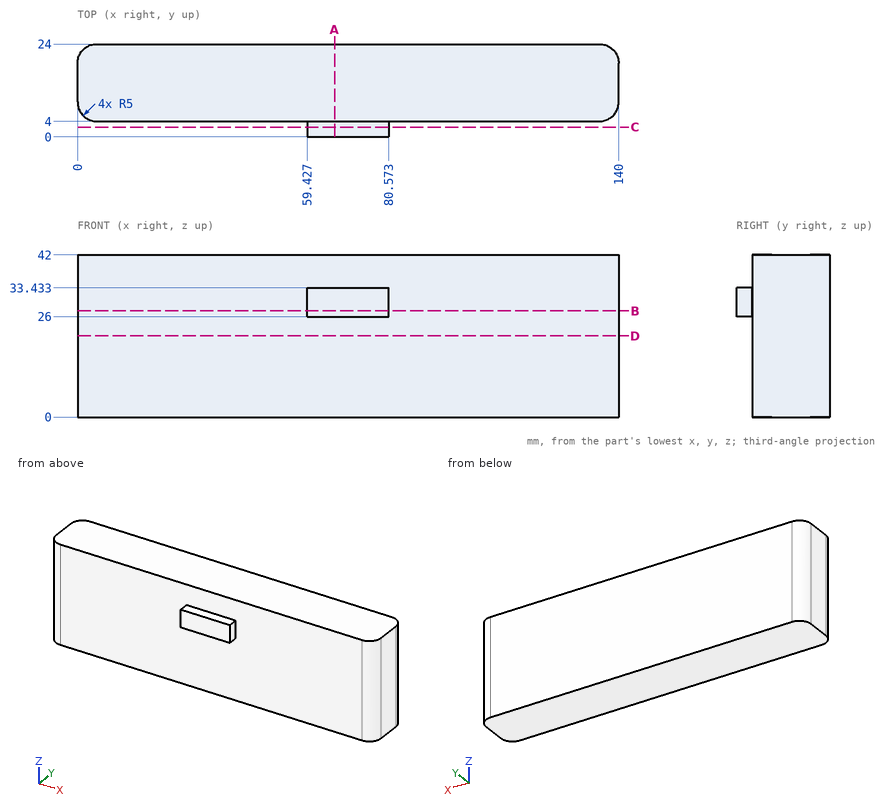
For this review, use the dimensioned drawing (mm, ordinates from the lowest corner) and the shaded views. Give positions to 0.01 mm unless a question says otherwise; leave off trailing zeros. Write each loop counter-clockwise with the first axis right and the second up, starting at its lowest first coordinate (ties: lowest second). Pieces come first, ordered by that corner, then holes. Notation, with made-up numbers: M 13,87 L 62,87 A15 cw 62,99 Z; hole C -34,42.5 d2. An arc over 180 degrees is marked long. Answer as a JSON object with one key per item and string values. Group by question number.
1) Clearance check with flat-ended pins moving along their axes: pin 1 Ø10 at (x, z) = (75, 7) entering from -Y; pin 2 Ø2 at (x, y) = (69, 2) entering from +Z; pin 3 Ø4.5 at (y, z) = (2.5, 30) entering from -X (1 decimal). State where each tip first meets the part, or that it passes through.
2) We need section D-D (z = 21). Give the boundary of the cut face in (x, y).
3) We need section A-A (x = 66.5). Give the boundary of the cut face in (y, z).
4) We need section C-C (y = 2.5). Give the boundary of the cut face in (x, z).
5) For line 1 along Y through (x, z) = (48.5, 19); line 2 along X through (y, z) = (8.5, 23.5) (1 decimal); line 3 along X through (y, z) = (4.5, 24.5) (1 decimal), list the stretches that pass through material, from the lowest coordinate up.
6) We need section B-B (z = 27.5). Give the boundary of the cut face in (x, y).
Answer key:
{
 "1": {"pin 1": "stops at y = 4", "pin 2": "stops at z = 33.43", "pin 3": "stops at x = 2.4"},
 "2": {"outline": "M 0,9 A5 ccw 5,4 L 135,4 A5 ccw 140,9 L 140,19 A5 ccw 135,24 L 5,24 A5 ccw 0,19 Z"},
 "3": {"outline": "M 0,26 L 4,26 L 4,0 L 24,0 L 24,42 L 4,42 L 4,33.43 L 0,33.43 Z"},
 "4": {"outline": "M 59.43,26 L 80.57,26 L 80.57,33.43 L 59.43,33.43 Z"},
 "5": {"line 1": "y = 4 to 24", "line 2": "x = 0 to 140", "line 3": "x = 2.8 to 137.2"},
 "6": {"outline": "M 0,9 A5 ccw 5,4 L 59.43,4 L 59.43,0 L 80.57,0 L 80.57,4 L 135,4 A5 ccw 140,9 L 140,19 A5 ccw 135,24 L 5,24 A5 ccw 0,19 Z"}
}
